Design review of the part built by this model. Coordinates are the model's own, in mm. A direction names the side the tool comes from. Give positions to 0.01 mm unless a question says otherwise; leave off trailing zeros. Write each loop counter-clockwise with the first axis right and the second up, starting at its lowest first coordinate (ties: lowest second). Pieces come first, ordered by that corner, then holes. Notation, with made-up numbers: M -30,-6 L 11,-6 A21 ccw 11,7 Z; hole C 82.25,85 d11. An arc over 180 degrees is marked long. Answer in a Markdown table with one row per item.
```python
from build123d import *

# Parameters (mm, degrees)
F0_W     = 100
F0_H     = 18
F1_DEPTH = 3
F2_R     = 5
F3_DEPTH = 1.5
F4_DEPTH = 1.5


with BuildPart() as f1:
    # F0 (on Top) → F1 (new body)
    with BuildSketch(Plane.XY):
        Rectangle(F0_W, F0_H)
        with BuildLine():
            ThreePointArc((-36.138195, -2.75), (-42.125, 0), (-36.138195, 2.75))
            Line((-36.138195, 2.75), (-24.124733, 1.996073))
            ThreePointArc((-24.124733, 1.996073), (-22.79217, 1.369209), (-22.25, 0))
            ThreePointArc((-22.25, 0), (-22.79217, -1.369209), (-24.124733, -1.996073))
            Line((-24.124733, -1.996073), (-36.138195, -2.75))
        make_face(mode=Mode.SUBTRACT)
        with BuildLine():
            ThreePointArc((36.138195, 2.75), (40.013123, 3.294098), (42.125, 0))
            ThreePointArc((42.125, 0), (40.013123, -3.294098), (36.138195, -2.75))
            Line((36.138195, -2.75), (24.124733, -1.996073))
            ThreePointArc((24.124733, -1.996073), (22.25, 0), (24.124733, 1.996073))
            Line((24.124733, 1.996073), (36.138195, 2.75))
        make_face(mode=Mode.SUBTRACT)
    extrude(amount=F1_DEPTH)

    # F2
    f2_edges = [f1.edges().sort_by_distance(p)[0] for p in [
        (-50, 9, 1.5),
        (-50, -9, 1.5),
        (50, 9, 1.5),
        (50, -9, 1.5),
    ]]
    fillet(f2_edges, radius=F2_R)

    # F0 (on Top) → F3 (join)
    with BuildSketch(Plane.XY):
        with BuildLine():
            ThreePointArc((-36.138195, 2.75), (-35.205902, 1.513123), (-34.875, 0))
            ThreePointArc((-34.875, 0), (-35.205902, -1.513123), (-36.138195, -2.75))
            Line((-36.138195, -2.75), (-24.124733, -1.996073))
            ThreePointArc((-24.124733, -1.996073), (-26.25, 0), (-24.124733, 1.996073))
            Line((-24.124733, 1.996073), (-36.138195, 2.75))
        make_face()
        with BuildLine():
            ThreePointArc((-22.25, 0), (-22.79217, 1.369209), (-24.124733, 1.996073))
            ThreePointArc((-24.124733, 1.996073), (-26.25, 0), (-24.124733, -1.996073))
            ThreePointArc((-24.124733, -1.996073), (-22.79217, -1.369209), (-22.25, 0))
        make_face()
    extrude(amount=F3_DEPTH)

    # F0 (on Top) → F4 (join)
    with BuildSketch(Plane.XY):
        with BuildLine():
            ThreePointArc((36.138195, -2.75), (34.875, 0), (36.138195, 2.75))
            Line((36.138195, 2.75), (24.124733, 1.996073))
            ThreePointArc((24.124733, 1.996073), (25.619209, 1.45783), (26.25, 0))
            ThreePointArc((26.25, 0), (25.619209, -1.45783), (24.124733, -1.996073))
            Line((24.124733, -1.996073), (36.138195, -2.75))
        make_face()
        with BuildLine():
            ThreePointArc((26.25, 0), (25.619209, 1.45783), (24.124733, 1.996073))
            ThreePointArc((24.124733, 1.996073), (22.25, 0), (24.124733, -1.996073))
            ThreePointArc((24.124733, -1.996073), (25.619209, -1.45783), (26.25, 0))
        make_face()
    extrude(amount=F4_DEPTH)


solid = f1.part
```
1) To check wall thickness, follow probe 1 along X at (y, z) = (0, 1.85) (3 decimals); probe 2 along Y at (x, z) = (-38.5, 0.95) (3 decimals); probe 3 along X at (y, z) = (1.75, 0.9). State the ranges of each line that lie inside material, in increasing order. Write a range as [from, to].
Geometry says:
| item | result |
|---|---|
| probe 1 | [-50, -42.125], [-22.25, 22.25], [42.125, 50] |
| probe 2 | [-9, -3.625], [3.625, 9] |
| probe 3 | [-50, -41.67], [-35.33, 35.33], [41.67, 50] |
2) Add section B-B (y = 7.25). Write out the cut boundary in (x, z).
Geometry says:
| item | result |
|---|---|
| outline | M -48.8,0 L 48.8,0 L 48.8,3 L -48.8,3 Z |
3) For faces 5 (the face through (29, 0, 1.5)), 6 (the face through (-1, 0, 3)), list the 3-axis set-ups (+Z, -Z, +X, -X, +Y, -Y) from which the entire face can be reached by the end or side of a thin tool; tool diameter is ignored.
Geometry says:
| item | result |
|---|---|
| face 5 | +Z |
| face 6 | +Z, +X, -X, +Y, -Y |
4) Insertion check: P1, Ø6, axis at x = -32, y = 1.5, coming from the +Z side; P2, Ø3, axis at x = 28, y = 0, coming from the +Z side; P3, Ø1.5, axis at y = -6.5, z = 2.5, coming from the +X side. Each pin has a flat end and moves straight along its axis. Give the tip position at first contact, or say it passes through.
Geometry says:
| item | result |
|---|---|
| P1 | z = 3 |
| P2 | z = 1.5 |
| P3 | x = 49.68 |
5) Add section A-A (x = -27). Write out the cut boundary in (y, z), and give its area (3 significant figures).
Geometry says:
| item | result |
|---|---|
| outline | M -9,0 L 9,0 L 9,3 L 2.18,3 L 2.18,1.5 L -2.18,1.5 L -2.18,3 L -9,3 Z |
| area | 47.5 mm^2 |
6) The part is to be moulded in two halves that separate along Y. For faces 1 (the face through (-1, -9, 1)), 2 (the face through (22.25, -0.04, 2.24)), 3 (the face through (50, 0, 1)), 4 (the face through (48, 8, 2)), say which applies: released by +Y, released by -Y, zero draft, split by the parting line, or undercut.
Geometry says:
| item | result |
|---|---|
| face 1 | released by -Y |
| face 2 | undercut |
| face 3 | zero draft |
| face 4 | released by +Y |
